Here's how the part is built. I have some questions about the finished solid (model axes, mm). A direction names the side the tool comes from. Round coordinates to 2 decimals unless told otherwise and drop trailing zeros. Write each loop counter-clockwise with the first axis right and the second up, starting at its lowest first coordinate (ties: lowest second). Pieces come first, ordered by that corner, then holes. Notation, with made-up numbers: (-13, 74) - (11, 74) arc R21 cw to (11, 86) - close; hole circle Ø5 at (-36.5, 29.5). An arc over 180 degrees is marked (long way). One line per question, with ' | ' between items. Start each with the question number.
(1) For faces 1 (the cylindrical face through (-11.014, 3.221, 5.925)), 2 (the flat face through (0, 0, 0)), 3 (the cylindrical face through (5.38, -27.07, 141.43)), which set-ups out of +Z, -Z, +X, -X, +Y, -Y let a thin tool reach every point of the face, with its end or its side?
(2) Imagine slicing it at B-B (z = 5). Write out the boundary of the cut face in (x, y) (3 decimals).
(3) Thinking about a two-plate mould opening in X: for faces 4 (the flat face through (0, -1, -2)), 5 (the flat face through (-10, 5, 54)), 6 (the cylindrical face through (-8.844, -27.07, 141.11)), which applies, pulls with the +X half, pulls with the -X half, needs draft (parallel to the pull), parting line crosses it, or undercut?
(4) Imagine slicing it at C-C (x = -8.5). Write out the boundary of the cut face in (y, z), plus the area to 3 significant figures.
(5) If I drill on L1, parallel to Z at x = 0, y = -28.5; L2, parallel to Y at x = 0, z = 110.55, over which ranges is the centre line in solid material (lowest first)?
(6) Will these pins go through, and if not, where does the flat tip stop? pin 1 (1.5 mm diameter, centred on x = 0.5, z = 82, fed in from -Y); pin 2 (12 mm diameter, centred on x = -7.5, z = 67, fed in from -Y); pin 3 (2 mm diameter, centred on x = -9, z = 114.5, fed in from -Y).
(7) Imagine slicing it at A-A (x = 4). Write out the boundary of the cut face in (y, z), plus the area to 3 significant figures.
from build123d import *
from build123d.topology import SkipClean

# Parameters (mm, degrees)
BOSS_EXTRUDE1_DEPTH = 110
BOSS_EXTRUDE3_START = -112
BOSS_EXTRUDE3_DEPTH = 2
SKETCH15_R          = 2.005
CUT_EXTRUDE1_DEPTH  = 2
SKETCH18_R          = 12
SKETCH18_R_2        = 10


with BuildPart() as part:
    # Sketch1 → Boss-Extrude1 (new body)
    with BuildSketch(Plane.XY):
        with BuildLine():
            Line((-10, 0), (-10, 10))
            Line((-10, 10), (-12, 10))
            Line((-12, 10), (-12, 0))
            ThreePointArc((-12, 0), (0, -12), (12, 0))
            Line((12, 0), (12, 10))
            Line((12, 10), (10, 10))
            Line((10, 10), (10, 0))
            ThreePointArc((10, 0), (0, -10), (-10, 0))
        make_face()
    extrude(amount=BOSS_EXTRUDE1_DEPTH)

    # Sketch8 → Boss-Extrude3 (add)
    with BuildSketch(Plane.XY.offset(110).offset(BOSS_EXTRUDE3_START)):
        with BuildLine():
            Line((-12, 10), (12, 10))
            Line((12, 10), (12, 0))
            ThreePointArc((12, 0), (0, -12), (-12, 0))
            Line((-12, 0), (-12, 10))
        make_face()
    extrude(amount=BOSS_EXTRUDE3_DEPTH)

    # Sketch15 → Cut-Extrude1 (cut)
    with BuildSketch(Plane.ZY.offset(12)):
        with Locations((5, 5)):
            Circle(SKETCH15_R)
    extrude(amount=-CUT_EXTRUDE1_DEPTH, mode=Mode.SUBTRACT)

    # Sweep2: sweep along a path in Sketch17
    with SkipClean():  # the faces are left unmerged after this step: merging them gives an invalid solid
        with BuildLine(Plane(origin=(0, 0, 0), x_dir=(0, 0, -1), z_dir=(1, 0, 0))) as sweep2_path:
            Line((-110, -12), (-111, -12))
            ThreePointArc((-111, -12), (-118.071067812, -14.928932188), (-121, -22))
            Line((-121, -22), (-121, -32))
        # Sketch18 → Sweep2 (sweep)
        with BuildSketch(Plane.XY.offset(110)):
            Circle(SKETCH18_R)
            Circle(SKETCH18_R_2, mode=Mode.SUBTRACT)
        sweep(path=sweep2_path.line)


solid = part.part
Check sheet entries:
1) face 1: -X | face 2: +Y | face 3: -Y
2) outline: (-12, 0) arc R12 ccw to (12, 0) - (12, 10) - (10, 10) - (10, 0) arc R10 cw to (-10, 0) - (-10, 2.995) - (-12, 2.995) - close; (-12, 7.005) - (-10, 7.005) - (-10, 10) - (-12, 10) - close
3) face 4: needs draft | face 5: undercut | face 6: parting line crosses it
4) outline: (-32, 124.53) - (-22, 124.53) arc R13.53 cw to (-8.47, 111) - (-8.47, -2) - (10, -2) - (10, 0) - (-5.27, 0) - (-5.27, 111) arc R16.73 ccw to (-22, 127.73) - (-32, 127.73) - close; (-32, 138.27) - (-22, 138.27) arc R27.27 cw to (5.27, 111) - (5.27, 110) - (8.47, 110) - (8.47, 111) arc R30.47 ccw to (-22, 141.47) - (-32, 141.47) - close | area: 681 mm^2
5) L1: 121 to 123, 143 to 145 | L2: -12 to -10, 10 to 12
6) pin 1: y = -12 | pin 2: y = -11.91 | pin 3: y = -9.47
7) outline: (-32, 121.69) - (-22, 121.69) arc R10.69 cw to (-11.31, 111) - (-11.31, -2) - (10, -2) - (10, 0) - (-9.17, 0) - (-9.17, 111) arc R12.83 ccw to (-22, 123.83) - (-32, 123.83) - close; (-32, 142.17) - (-22, 142.17) arc R31.17 cw to (9.17, 111) - (9.17, 110) - (11.31, 110) - (11.31, 111) arc R33.31 ccw to (-22, 144.31) - (-32, 144.31) - close | area: 475 mm^2
